```python
from build123d import *

# Parameters (mm, degrees)
F0_W     = 30
F0_H     = 30
F1_DEPTH = 11
F2_W     = 26
F2_H     = 30
F3_DEPTH = 9
F4_W     = 1.45
F4_H     = 15
F5_DEPTH = 11
F6_W     = 10.1
F6_H     = 15
F7_DEPTH = 2.5
F8_W     = 3.5
F8_H     = 2.5
F9_DEPTH = 13.001
F10_R    = 1


with BuildPart() as f1:
    # F0 (on Top) → F1 (new body)
    with BuildSketch(Plane.XY):
        Rectangle(F0_W, F0_H)
    extrude(amount=F1_DEPTH)

    # F2 (on face) → F3 (cut)
    with BuildSketch(Plane(origin=(0, 0, 0), x_dir=(1, 0, 0), z_dir=(0, 0, -1))):
        Rectangle(F2_W, F2_H)
    extrude(amount=-F3_DEPTH, mode=Mode.SUBTRACT)

    # F4 (on face) → F5 (join)
    with BuildSketch(Plane.XY.offset(11)):
        with Locations((-14.275, 0)):
            Rectangle(F4_W, F4_H)
        with Locations((-2.725, 0)):
            Rectangle(F4_W, F4_H)
    extrude(amount=F5_DEPTH)

    # F6 (on face) → F7 (join)
    with BuildSketch(Plane.XY.offset(11)):
        with Locations((-8.5, 0)):
            Rectangle(F6_W, F6_H)
    extrude(amount=F7_DEPTH)

    # F8 (on face) → F9 (cut, through all)
    with BuildSketch(Plane.YZ.offset(-2)):
        with Locations((-4.25, 12.25)):
            Rectangle(F8_W, F8_H)
        with Locations((4.25, 12.25)):
            Rectangle(F8_W, F8_H)
    extrude(amount=-F9_DEPTH, mode=Mode.SUBTRACT)

    # F10
    f10_edges = [f1.edges().sort_by_distance(p)[0] for p in [
        (-14.275, 7.5, 22),
        (-14.275, -7.5, 22),
        (-2.725, -7.5, 22),
        (-2.725, 7.5, 22),
        (-15, -11.25, 11),
        (-15, 11.25, 11),
        (-15, 4.25, 11),
        (-15, -4.25, 11),
        (15, 0, 11),
        (-14, -15, 0),
        (14, -15, 0),
        (-14, 15, 0),
        (14, 15, 0),
    ]]
    fillet(f10_edges, radius=F10_R)


solid = f1.part
```
Work out the finished part from the listing and answer in its coordinate system (mm). A direction names the side the tool comes from. Give positions to 0.01 mm unless a question says otherwise; leave off trailing zeros. Loops run counter-clockwise (first coordinate to the right, second up) from the corner with the lowest first, then second, coordinate; pieces in that order, holes last. Notation, with made-up numbers: (30, 70.25) - (76, 70.25) arc R24 ccw to (76, 101.25) - close; hole circle Ø8 at (31.5, 28). An arc over 180 degrees is marked (long way). Use CSV: the item, a comma, the result in double quotes. Start each with the question number.
(1) Find section C-C, the plane x = -7.5. Determine the outline of the cut face in (y, z).
(2) A tool of negligible diameter and unlimited length cuts with its end or side. For faces 4 (the face through (-2, 0, 16)), 5 (the face through (-9, 0, 13.5)), 6 (the face through (-3, -4, 13.5)), 7 (the face through (-14.699, -11.198, 10.715)), from which of +Z, -Z, +X, -X, +Y, -Y can it reach the whole face along a straight path? Write none if from no direction.
(3) Each of these flat-tipped pins is pushed along its axis until it touches: pin 1 (1.5 mm diameter, centred on x = -8, y = 0.5, fed in from +Z); pin 2 (5 mm diameter, centred on x = -1, y = 8, fed in from -Z); pin 3 (1.8 mm diameter, centred on x = -9.5, z = 12, fed in from -Y); pin 4 (2 mm diameter, centred on x = -3, z = 7.5, fed in from -Y). Where does it stop, or does it pass through?
(4) Find section D-D, the plane z = 15.75. Determine the outline of the cut face in (x, y).
(5) Determine the mould class of faces 1 (the face through (-14, 4, 13.5)), 2 (the face through (-13, 0, 4)), 3 (the face through (-9, -7, 13.5)) for opening direction Z: released by +Z, released by -Z, zero draft, split by the parting line, or undercut.
(6) Find section B-B, the plane y = -3.5. Determine the outline of the cut face in (x, z), plus the area to 3 significant figures.
(7) Find section A-A, the plane z = 2.75. Determine the outline of the cut face in (x, y).
(8) Find the intervals of material crossed by L1, parallel to X at y = 1, z = 19.75; L2, parallel to X at y = -4.75, z = 2.5; L3, parallel to Z at x = 12, y = 3, in increasing order.
Results found:
1,outline,"(-15, 9) - (15, 9) - (15, 11) - (7.5, 11) - (7.5, 13.5) - (6, 13.5) - (6, 11) - (2.5, 11) - (2.5, 13.5) - (-2.5, 13.5) - (-2.5, 11) - (-6, 11) - (-6, 13.5) - (-7.5, 13.5) - (-7.5, 11) - (-15, 11) - close"
2,face 4,"+Z, +X, +Y, -Y"
2,face 5,"+Z, +Y, -Y"
2,face 6,"+X, -X"
2,face 7,"+Z, -X, -Y"
3,pin 1,"z = 13.5"
3,pin 2,"z = 9"
3,pin 3,"y = -7.5"
3,pin 4,"through"
4,outline,"(-15, -7.5) - (-13.55, -7.5) - (-13.55, 7.5) - (-15, 7.5) - close; (-3.45, -7.5) - (-2, -7.5) - (-2, 7.5) - (-3.45, 7.5) - close"
5,face 1,"undercut"
5,face 2,"zero draft"
5,face 3,"released by +Z"
6,outline,"(-15, 0) - (-13, 0) - (-13, 9) - (13, 9) - (13, 0) - (15, 0) - (15, 10) arc R1 ccw to (14, 11) - (-14, 11) arc R1 ccw to (-15, 10) - close; (-15, 13.5) - (-13.55, 13.5) - (-13.55, 22) - (-15, 22) - close; (-3.45, 13.5) - (-2, 13.5) - (-2, 22) - (-3.45, 22) - close"
6,area,"120 mm^2"
7,outline,"(-15, -15) - (-13, -15) - (-13, 15) - (-15, 15) - close; (13, -15) - (15, -15) - (15, 15) - (13, 15) - close"
8,L1,"-15 to -13.55, -3.45 to -2"
8,L2,"-15 to -13, 13 to 15"
8,L3,"9 to 11"
